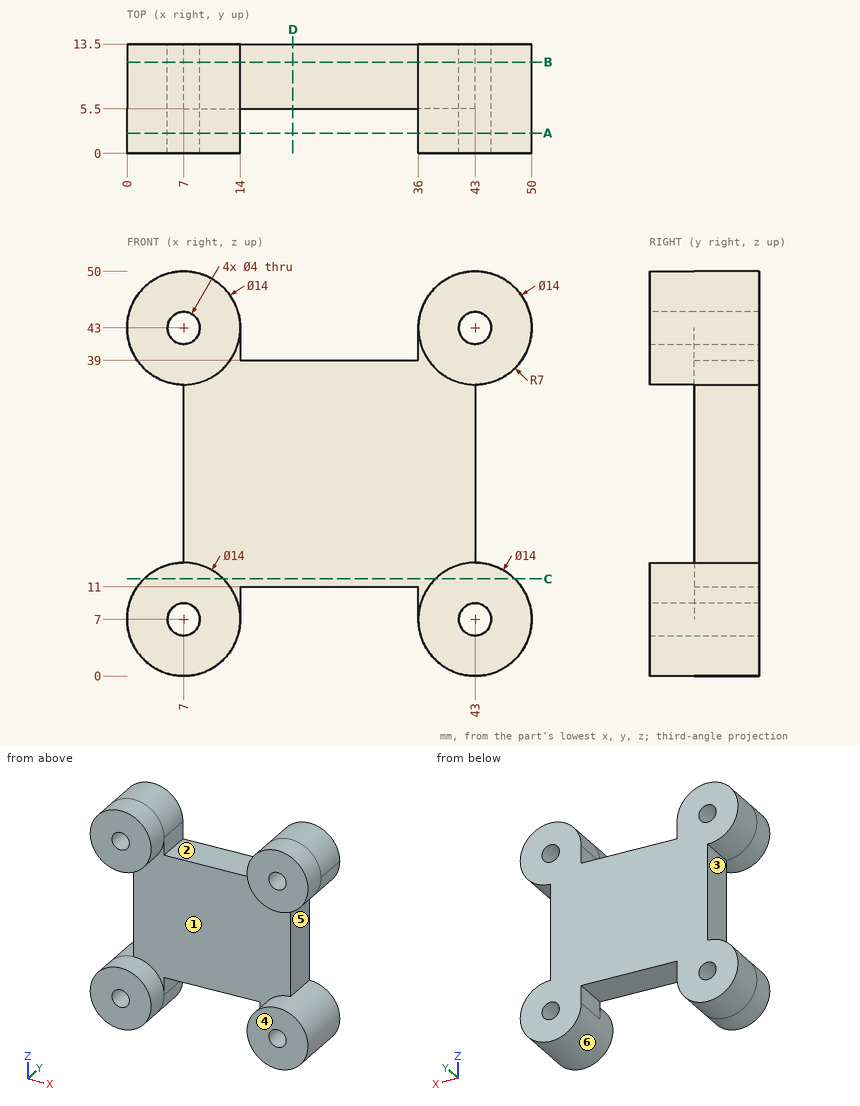
Geometry check sheet. Reference: drawing and pictorial views, mm from the part's lowest x, y, z. A direction names the side the tool comes from. Give positions to 0.01 mm unless a question says otherwise; leave off trailing zeros. Order: outer loops, then holes, each group sorted by start corner. A loop starts at its lowest first (then second) coordinate and runs counter-clockwise, first axis right, second up. Notation, with made-up numbers: M 1,37 L 7,37 A35 ccw 7,70 Z; hole C -31,-4.75 d10. An arc over 180 degrees is marked long. Answer in a Markdown table with one row per item. Add a question column.
Q1. Sectioned sample at D-D, the plane x = 20.5. Record the boundary of the cut face in (y, z).
Q2. Sectioned sample at B-B, the plane y = 11.25. Record the boundary of the cut face in (x, z).
Q3. Thickness scan on L1, parallel to X at y = 8.5, z = 7; L2, parallel to Z at x = 44, y = 4.25. Record the ranges inside material, lowest first.
Q4. Sectioned sample at A-A, the plane y = 2.5. Record the boundary of the cut face in (x, z).
Q5. Sectioned sample at C-C, the plane z = 12. Record the boundary of the cut face in (x, y), and give its area (3 significant figures).
Q6. Access from +Z, -Z, +X, -X, +Y, -Y to the whole of each face (thin tool, end or side, straight path). Record for the marked faces 1, 2 and 3.
Q7. Release check for a two-part mould opening along X. For the marked faces 4, 5 and 6 record: released by +X, released by -X, zero draft, split by the parting line, or undercut.
Q8. Gauge pin test, flat ends, axial feed: pin 1 Ø5 at (x, y) = (18, 5) entering from -Z; pin 2 Ø3 at (y, z) = (8, 9) entering from +X; pin 3 Ø6.5 at (y, z) = (9.5, 30) entering from +X. Record the tip position at first contact, or that the pin passes through.
Verdict:
| question | item | result |
|---|---|---|
| 1 | outline | M 5.5,11 L 13.5,11 L 13.5,39 L 5.5,39 Z |
| 2 | outline | M 7,14 A7 ccw long 14,7 L 14,11 L 36,11 L 36,7 A7 ccw long 43,14 L 43,36 A7 ccw long 36,43 L 36,39 L 14,39 L 14,43 A7 ccw long 7,36 Z; hole C 7,7 d4; hole C 7,43 d4; hole C 43,7 d4; hole C 43,43 d4 |
| 3 | L1 | 0 to 5, 9 to 14, 36 to 41, 45 to 50 |
| 3 | L2 | 0.07 to 5.27, 8.73 to 13.93, 36.07 to 41.27, 44.73 to 49.93 |
| 4 | outline | C 7,7 d14; C 7,43 d14; C 43,7 d14; C 43,43 d14; hole C 7,7 d4; hole C 7,43 d4; hole C 43,7 d4; hole C 43,43 d4 |
| 5 | outline | M 2.1,0 L 11.9,0 L 11.9,5.5 L 38.1,5.5 L 38.1,0 L 47.9,0 L 47.9,13.5 L 2.1,13.5 Z |
| 5 | area | 474 mm² |
| 6 | face 1 | -Y |
| 6 | face 2 | +Z, +Y, -Y |
| 6 | face 3 | -X, +Y, -Y |
| 7 | face 4 | zero draft |
| 7 | face 5 | released by +X |
| 7 | face 6 | undercut |
| 8 | pin 1 | z = 11 |
| 8 | pin 2 | x = 49.98 |
| 8 | pin 3 | x = 43 |
